Check sheet for the modelled part. Datum: model origin and axes. Units: mm. Round coordinates to 2 decimals unless told otherwise and drop trailing zeros. Loops run counter-clockwise (first coordinate to the right, second up) from the corner with the lowest first, then second, coordinate; pieces in that order, holes last. Notation, with made-up numbers: M 14.5,12 L 47.5,12 A15 ccw 47.5,28 Z; hole C 48,87.25 d11. An arc over 180 degrees is marked long. Write item = value, one per line. Start each with the question number.
(1) Cross-section at A-A on z = 142. Record the boundary of the cut face in (x, y).
(2) Mould release check, pull along Y, two halves, no side actions. Record for faces 1 (the face through (5, 11, 124)), 2 (the face through (2, 59.908, 123)), 3 (the face through (2.46, -6.86, 133.92)): pulls with the +Y half, pulls with the -Y half, needs draft (parallel to the pull), parting line crosses it, or undercut.
(3) Cross-section at C-C on z = 159. Record the boundary of the cut face in (x, y), plus the area to 4 significant figures.
(4) Scan lines: L1, parallel to Y at x = 1.75, z = 148; L2, parallel to Y at x = 3.45, z = 142; L3, parallel to Y at x = 1, z = 135. Record each from-to range of solid material in increasing order. Write a range as from..to.
(5) Cross-section at B-B on x = 1. Record the boundary of the cut face in (y, z), plus the area to 3 significant figures.
from build123d import *

# Parameters (mm, degrees)
SKIZZE1_R                       = 11.5
SKIZZE1_R_2                     = 2.25
SKIZZE1_R_3                     = 2.05
AUFSATZ_LINEAR_AUSTRAGEN1_DEPTH = 5
VERRUNDUNG1_R                   = 1


with BuildPart() as part:
    # Skizze1 → Aufsatz-Linear austragen1 (new body)
    with BuildSketch(Plane(origin=(0, 0, 0), x_dir=(0, 0, -1), z_dir=(1, 0, 0))):
        Polygon((-92, 59.908196572), (-192, 59.908196572), (-192, -40.091803428), (-92, -40.091803428), (-55, -40.091803428), (-55, 59.908196572), align=None)
        with Locations((-142, 9.908196572)):
            Circle(SKIZZE1_R, mode=Mode.SUBTRACT)
        with Locations((-148, 25.814170293)):
            Circle(SKIZZE1_R_2, mode=Mode.SUBTRACT)
        with Locations((-136, 25.814170293)):
            Circle(SKIZZE1_R_2, mode=Mode.SUBTRACT)
        with Locations((-159, 9.908196572)):
            Circle(SKIZZE1_R_3, mode=Mode.SUBTRACT)
        with Locations((-148, -5.997777148)):
            Circle(SKIZZE1_R_2, mode=Mode.SUBTRACT)
        with Locations((-136, -5.997777148)):
            Circle(SKIZZE1_R_2, mode=Mode.SUBTRACT)
    extrude(amount=AUFSATZ_LINEAR_AUSTRAGEN1_DEPTH)

    # Verrundung1
    verrundung1_edges = [part.edges().sort_by_distance(p)[0] for p in [
        (2.5, 59.908196572, 192),
        (2.5, 59.908196572, 55),
        (2.5, -40.091803428, 55),
        (2.5, -40.091803428, 192),
    ]]
    fillet(verrundung1_edges, radius=VERRUNDUNG1_R)


solid = part.part
Result:
q1.outline = M 0,-40.09 L 5,-40.09 L 5,-1.59 L 0,-1.59 Z; M 0,21.41 L 5,21.41 L 5,59.91 L 0,59.91 Z
q2.face_1 = needs draft
q2.face_2 = pulls with the +Y half
q2.face_3 = undercut
q3.outline = M 0,-40.09 L 5,-40.09 L 5,7.86 L 0,7.86 Z; M 0,11.96 L 5,11.96 L 5,59.91 L 0,59.91 Z
q3.area = 479.5 mm^2
q4.L1 = -40.09..-8.25, -3.75..0.1, 19.72..23.56, 28.06..59.91
q4.L2 = -40.09..-1.59, 21.41..59.91
q4.L3 = -40.09..-8.01, -3.98..0.78, 19.03..23.8, 27.83..59.91
q5.outline = M -40.09,56 A1 ccw -39.09,55 L 58.91,55 A1 ccw 59.91,56 L 59.91,191 A1 ccw 58.91,192 L -39.09,192 A1 ccw -40.09,191 Z; hole C -6,136 d4.5; hole C -6,148 d4.5; hole C 9.91,142 d23; hole C 9.91,159 d4.1; hole C 25.81,136 d4.5; hole C 25.81,148 d4.5
q5.area = 13,200 mm^2
